Verification items for the finished model (mm, model axes). Coordinates: 2 decimals unless noted, no trailing zeros. Write each loop counter-clockwise with the first axis right and the second up, starting at its lowest first coordinate (ties: lowest second). Pieces come first, ordered by that corner, then holes. Notation, with made-up numbers: M 62,-34.75 L 73,-34.75 A19 ccw 73,-4.75 Z; hole C -8.5,41 d4. An arc over 180 degrees is marked long. Answer in a Markdown table with one row per item.
from build123d import *

# Parameters (mm, degrees)
F1_DEPTH = 0.5
F2_D     = 6


with BuildPart() as f1:
    # F0 (on Right) → F1 (new body)
    with BuildSketch(Plane.YZ):
        with BuildLine():
            Line((49, -24.75), (49, 24.75))
            ThreePointArc((49, 24.75), (0, 73.75), (-49, 24.75))
            Line((-49, 24.75), (-49, -24.75))
            ThreePointArc((-49, -24.75), (0, -73.75), (49, -24.75))
        make_face()
        with BuildLine():
            ThreePointArc((-21, 2.977024), (0, 55), (21, 2.977024))
            Line((21, 2.977024), (21, -2.977024))
            ThreePointArc((21, -2.977024), (0, -55), (-21, -2.977024))
            Line((-21, -2.977024), (-21, 2.977024))
        make_face(mode=Mode.SUBTRACT)
    extrude(amount=F1_DEPTH)

    # F2 (through all)
    with Locations(Plane(origin=(0, 0, 0), x_dir=(0, 1, 0), z_dir=(-1, 0, 0))):
        with Locations((22, 59.347688), (-22, 59.347688), (-41, 21.75), (-41, -21.75), (-22, -59.347688), (22, -59.347688), (41, -21.75), (41, 21.75)):
            Hole(F2_D / 2)


solid = f1.part
1) Release check for a two-part mould opening along Z. For faces 1 (the face through (0.254, 43.997, -21.882)), 2 (the face through (0.25, 1.08, 73.74)), 3 (the face through (0.5, -22, 1)) record: +Z half, -Z half, draft (parallel to the pull), parting line (faces both ways), or undercut.
Response values:
| item | result |
|---|---|
| face 1 | undercut |
| face 2 | +Z half |
| face 3 | draft |
2) Sectioned sample at A-A (y = 0). Record the cut outline in (x, z), then the cut area to 4 significant figures.
Response values:
| item | result |
|---|---|
| outline | M 0,-73.75 L 0.5,-73.75 L 0.5,-55 L 0,-55 Z; M 0,55 L 0.5,55 L 0.5,73.75 L 0,73.75 Z |
| area | 18.75 mm² |
3) Sectioned sample at D-D (z = 27.5). Record the cut outline in (x, y).
Response values:
| item | result |
|---|---|
| outline | M 0,-48.92 L 0.5,-48.92 L 0.5,-30.12 L 0,-30.12 Z; M 0,30.12 L 0.5,30.12 L 0.5,48.92 L 0,48.92 Z |
4) Sectioned sample at B-B (z = -21.75). Record the cut outline in (x, y), then the cut area to 3 significant figures.
Response values:
| item | result |
|---|---|
| outline | M 0,-49 L 0.5,-49 L 0.5,-44 L 0,-44 Z; M 0,-38 L 0.5,-38 L 0.5,-30.1 L 0,-30.1 Z; M 0,30.1 L 0.5,30.1 L 0.5,38 L 0,38 Z; M 0,44 L 0.5,44 L 0.5,49 L 0,49 Z |
| area | 12.9 mm² |
5) Sectioned sample at C-C (y = -42). Record the cut outline in (x, z), then the cut area to 3 significant figures.
Response values:
| item | result |
|---|---|
| outline | M 0,-49.99 L 0.5,-49.99 L 0.5,-24.58 L 0,-24.58 Z; M 0,-18.92 L 0.5,-18.92 L 0.5,18.92 L 0,18.92 Z; M 0,24.58 L 0.5,24.58 L 0.5,49.99 L 0,49.99 Z |
| area | 44.3 mm² |
6) Thickness scan on L1, parallel to Y at x = 0.3, z = -21.75; L2, parallel to Z at x = 0.2, y = -22; L3, parallel to Z at x = 0.2, y = 40. Record the ranges inside material, lowest first. Write a range as [from, to].
Response values:
| item | result |
|---|---|
| L1 | y = [-49, -44], [-38, -30.1], [30.1, 38], [44, 49] |
| L2 | z = [-68.53, -62.35], [-56.35, -45.51], [-3.99, 3.99], [45.51, 56.35], [62.35, 68.53] |
| L3 | z = [-53.05, -24.58], [-18.92, 18.92], [24.58, 53.05] |
7) Depth check by flat-ended pin: pin 1 (5 mm diameter, centred on y = -41, z = 21.75, fed in from -X). Enter the tip coordinate at first touch or a pass-through.
Response values:
| item | result |
|---|---|
| pin 1 | passes through |
